The figure shows three views and two pictorial views of one solid part (mm, origin at its lowest corner). Answer the questions. A direction names the side the tool comes from. Give positions to 0.01 mm unless a question says otherwise; leave off trailing zeros. Loops run counter-clockwise (first coordinate to the right, second up) from the corner with the lowest first, then second, coordinate; pieces in that order, holes last.
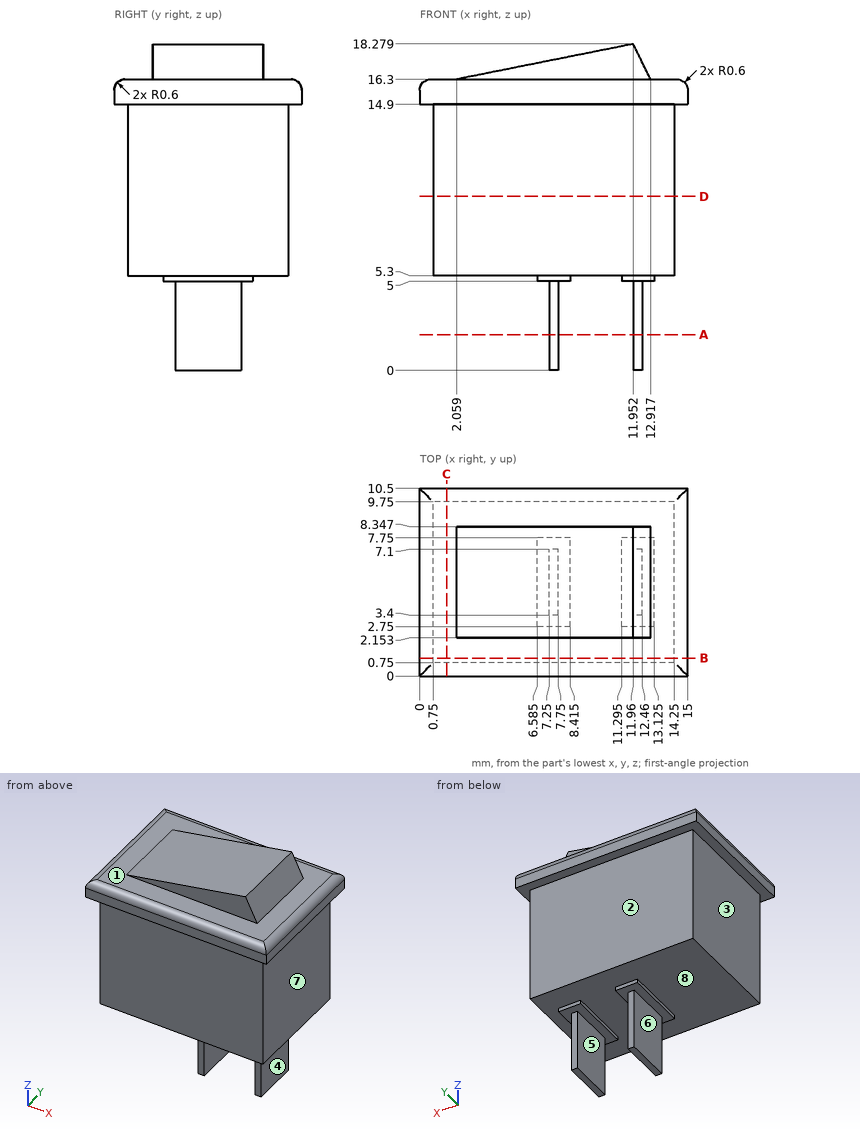
Q1. Section C-C on x = 1.5 is taken. Give the vertices of the cut face in (y, z), plus the area to 3 significant figures.
Q2. Given pin 1 (1 mm diameter, centred on x = 8, y = 3.5, fed in from +Z); pin 2 (0.6 mm diameter, centred on x = 9.5, z = 17, fed in from -Y); pin 3 (1.5 mm diameter, centred on y = 1.5, z = 13, fed in from -X); pin 4 (6 mm diameter, centred on y = 8.5, z = 13.5, fed in from -X), each flat-ended and moving along its own axis, determine where each tip first touches the part or whether it passes through.
Q3. Section D-D on z = 9.75 is taken. Give the vertices of the cut face in (x, y), plus the area to 4 significant figures.
Q4. Consider line 1 along X through (y, z) = (4.5, 1.5); line 2 along Z through (x, y) = (10, 8.5); line 3 along Y through (x, z) = (14, 9.25). Determine where each line is inside the solid, lowest interval first.
Q5. Section B-B on y = 1 is taken. Give the vertices of the cut face in (x, z).
Q6. Determine the mould class of the marked faces 6, 7 and 8 for opening direction X: +X half, -X half, draft (parallel to the pull), parting line (faces both ways), or undercut.
Q7. Section A-A on z = 2 is taken. Give the vertices of the cut face in (x, y).
Q8. Which of the six approach directions +Z, -Z, +X, -X, +Y, -Y give full straight-line access (tool end or side, diameter ignored) to the marked faces 1, 2, 3, 4 and 5?
Check result:
1. outline: (0, 14.9) - (0.75, 14.9) - (0.75, 5.3) - (9.75, 5.3) - (9.75, 14.9) - (10.5, 14.9) - (10.5, 15.7) arc R0.6 ccw to (9.9, 16.3) - (0.6, 16.3) arc R0.6 ccw to (0, 15.7) - close
1. area: 101 mm2
2. pin 1: stops at z = 17.59
2. pin 2: stops at y = 2.15
2. pin 3: stops at x = 0.75
2. pin 4: stops at x = 0
3. outline: (0.75, 0.75) - (14.25, 0.75) - (14.25, 9.75) - (0.75, 9.75) - close
3. area: 121.5 mm2
4. line 1: x = 7.25 to 7.75, 11.96 to 12.46
4. line 2: z = 5.3 to 16.3
4. line 3: y = 0.75 to 9.75
5. outline: (0, 14.9) - (0.75, 14.9) - (0.75, 5.3) - (14.25, 5.3) - (14.25, 14.9) - (15, 14.9) - (15, 15.7) arc R0.6 ccw to (14.4, 16.3) - (0.6, 16.3) arc R0.6 ccw to (0, 15.7) - close
6. face 6: -X half
6. face 7: +X half
6. face 8: undercut
7. outline: (7.25, 3.4) - (7.75, 3.4) - (7.75, 7.1) - (7.25, 7.1) - close; (11.96, 3.4) - (12.46, 3.4) - (12.46, 7.1) - (11.96, 7.1) - close
8. face 1: +Z
8. face 2: -Z, +X, -X, +Y
8. face 3: -Z, -X, +Y, -Y
8. face 4: -Z, +X, +Y, -Y
8. face 5: -Z, +Y, -Y
